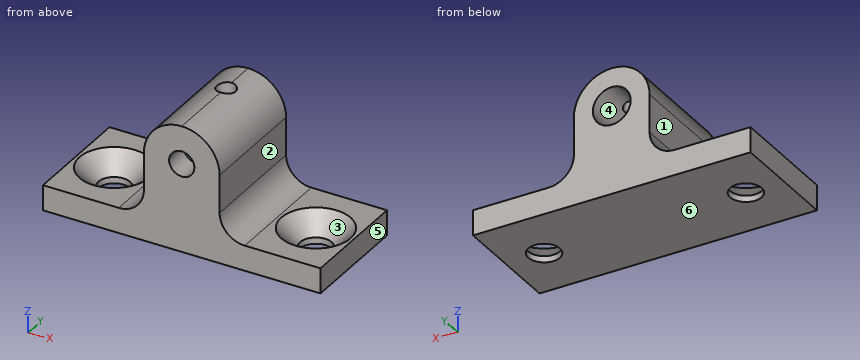
from build123d import *

# Parameters (mm, degrees)
F1_DEPTH       = 9
F3_D           = 2.5
F3_CSINK_D     = 5.5
F3_CSINK_ANGLE = 90
F5_D           = 2
F5_CBORE_D     = 3
F5_CBORE_DEPTH = 7
F8_D           = 1.5
F8_DEPTH       = 3
F8_START       = 0.0952626
F8_TIP         = 0.4506454643


with BuildPart() as f1:
    # F0 (on Front) → F1 (new body)
    with BuildSketch(Plane.XZ):
        with BuildLine():
            Line((0, 10), (0, 0))
            Line((0, 0), (11, 0))
            Line((11, 0), (11, 2))
            Line((11, 2), (5, 2))
            ThreePointArc((5, 2), (3.5857864376, 2.5857864376), (3, 4))
            Line((3, 4), (3, 7))
            ThreePointArc((3, 7), (2.1213203436, 9.1213203436), (0, 10))
        make_face()
    extrude(amount=F1_DEPTH)

    # F3 (through all)
    with Locations(Plane.XY.offset(2)):
        with Locations((8, -4.5)):
            CounterSinkHole(F3_D / 2, F3_CSINK_D / 2, counter_sink_angle=F3_CSINK_ANGLE)

    # F4: F1 across plane


with BuildPart() as f1_1:
    add(f1.part)
    add(f1.part.mirror(Plane.YZ))

    # F5 (through all)
    with Locations(Plane(origin=(0, 0, 0), x_dir=(1, 0, 0), z_dir=(0, 1, 0))):
        with Locations((0, -7)):
            CounterBoreHole(F5_D / 2, F5_CBORE_D / 2, F5_CBORE_DEPTH)

    # F8
    # its depths count from where the whole tool has entered the part; down to there all is cleared
    with Locations(Plane.XY.offset(10).offset(-F8_START)):
        with Locations((0, -3)):
            Hole(F8_D / 2, depth=F8_DEPTH)
            with Locations((0, 0, -(F8_DEPTH + F8_TIP / 2))):  # 118° drill point
                Cone(0, F8_D / 2, F8_TIP, mode=Mode.SUBTRACT)


solid = f1_1.part
Geometry check sheet. Reference: the model listing, model coordinates, mm. Face numbers are marked on the shaded views. A direction names the side the tool comes from. Round coordinates to 2 decimals unless told otherwise and drop trailing zeros. Order: outer loops, then holes, each group sorted by start corner. A loop starts at its lowest first (then second) coordinate and runs counter-clockwise, first axis right, second up. Notation, with made-up numbers: (-22.75, 6) -> (-0.75, 6) arc R17 cw to (-0.75, 30) -> close; hole circle Ø7 at (45.25, -28). An arc over 180 degrees is marked (long way). Use one line per item in the form item = value.
1. Cross-section at D-D, the plane z = 9. Enter the section's corners in (x, y).
Working result:
outline = (-2.24, -9) -> (2.24, -9) -> (2.24, 0) -> (-2.24, 0) -> close; hole circle Ø1.5 at (0, -3)
2. Cross-section at A-A, the plane y = -4.5. Enter the section's corners in (x, z), plus the area to 3 significant figures.
Working result:
outline = (-11, 0) -> (-9.25, 0) -> (-9.25, 0.5) -> (-10.75, 2) -> (-11, 2) -> close; (-6.75, 0) -> (6.75, 0) -> (6.75, 0.5) -> (5.25, 2) -> (5, 2) arc R2 cw to (3, 4) -> (3, 7) arc R3 ccw to (-3, 7) -> (-3, 4) arc R2 cw to (-5, 2) -> (-5.25, 2) -> (-6.75, 0.5) -> close; (9.25, 0) -> (11, 0) -> (11, 2) -> (10.75, 2) -> (9.25, 0.5) -> close; hole circle Ø3 at (0, 7)
area = 68.3 mm^2
3. Go/stop test with flat-tipped pins: pin 1 (1.5 mm diameter, centred on y = -3, z = 5, fed in from +X); pin 2 (1.5 mm diameter, centred on y = -4.5, z = 5, fed in from -X); pin 3 (3 mm diameter, centred on x = 6.5, y = -6, fed in from +Z). Record where each tip stops, or that it passes through.
Working result:
pin_1 = 3
pin_2 = -3
pin_3 = 2
4. Scan lines: line 1 along Y through (x, z) = (8, 0.3); line 2 along X through (y, z) = (-8, 7); line 3 along Z through (x, y) = (0, -7.8). Record each from-to range of solid material in increasing order. Write a range as from..to.
Working result:
line_1 = -9..-5.75, -3.25..0
line_2 = -3..-1, 1..3
line_3 = 0..6, 8..10
5. Cross-section at B-B, the plane x = -8. Enter the section's corners in (y, z), plus the area to 4 significant figures.
Working result:
outline = (-9, 0) -> (-5.75, 0) -> (-5.75, 0.5) -> (-7.25, 2) -> (-9, 2) -> close; (-3.25, 0) -> (0, 0) -> (0, 2) -> (-1.75, 2) -> (-3.25, 0.5) -> close
area = 10.75 mm^2
6. Cross-section at C-C, the plane x = 0.5. Enter the section's corners in (y, z), plus the area to 3 significant figures.
Working result:
outline = (-9, 0) -> (0, 0) -> (0, 5.59) -> (-7, 5.59) -> (-7, 6.13) -> (-9, 6.13) -> close; (-9, 7.87) -> (-7, 7.87) -> (-7, 8.41) -> (-3.56, 8.41) -> (-3.56, 9.96) -> (-9, 9.96) -> close; (-2.44, 8.41) -> (0, 8.41) -> (0, 9.96) -> (-2.44, 9.96) -> close
area = 64.6 mm^2
7. Set-up check for the marked faces 1, 2 and 3: record each of +Z, -Z, +X, -X, +Y, -Y from which the full face is reachable in a straight line by a thin tool's end or side.
Working result:
face_1 = +Z, -X, +Y, -Y
face_2 = +Z, +X, +Y, -Y
face_3 = +Z
8. Mould release check, pull along X, two halves, no side actions. Record for the marked faces 4, 5 and 6: pulls with the +X half, pulls with the -X half, needs draft (parallel to the pull), parting line crosses it, or undercut.
Working result:
face_4 = undercut
face_5 = pulls with the +X half
face_6 = needs draft
